from build123d import *

# Parameters (mm, degrees)
F0_W     = 355
F0_H     = 173
F0_R     = 3
F0_R_2   = 2.5
F0_R_3   = 3.25
F1_DEPTH = 20
F2_R     = 4
F3_DEPTH = 20


with BuildPart() as f1:
    # F0 (on Top) → F1 (new body)
    with BuildSketch(Plane.XY):
        with Locations((177.5, 86.5)):
            Rectangle(F0_W, F0_H)
        with Locations((29, 18)):
            Circle(F0_R, mode=Mode.SUBTRACT)
        with Locations((134.5, 72)):
            Circle(F0_R_2, mode=Mode.SUBTRACT)
        with BuildLine():
            Line((206, 13), (198, 13))
            ThreePointArc((198, 13), (196.585786, 13.585786), (196, 15))
            Line((196, 15), (196, 42))
            ThreePointArc((196, 42), (196.585786, 43.414214), (198, 44))
            Line((198, 44), (206, 44))
            ThreePointArc((206, 44), (207.414214, 43.414214), (208, 42))
            Line((208, 42), (208, 15))
            ThreePointArc((208, 15), (207.414214, 13.585786), (206, 13))
        make_face(mode=Mode.SUBTRACT)
        with Locations((269.5, 72)):
            Circle(F0_R_2, mode=Mode.SUBTRACT)
        with Locations((29, 88)):
            Circle(F0_R, mode=Mode.SUBTRACT)
        with BuildLine():
            Line((151.5, 121), (151.5, 71))
            ThreePointArc((151.5, 71), (150.328427, 68.171573), (147.5, 67))
            ThreePointArc((147.5, 67), (144.671573, 68.171573), (143.5, 71))
            Line((143.5, 71), (143.5, 121))
            ThreePointArc((143.5, 121), (144.671573, 123.828427), (147.5, 125))
            ThreePointArc((147.5, 125), (150.328427, 123.828427), (151.5, 121))
        make_face(mode=Mode.SUBTRACT)
        with Locations((134.5, 122)):
            Circle(F0_R_2, mode=Mode.SUBTRACT)
        with Locations((29, 158)):
            Circle(F0_R, mode=Mode.SUBTRACT)
        with BuildLine():
            Line((237, 51), (167, 51))
            ThreePointArc((167, 51), (159.928932, 53.928932), (157, 61))
            Line((157, 61), (157, 131))
            ThreePointArc((157, 131), (159.928932, 138.071068), (167, 141))
            Line((167, 141), (237, 141))
            ThreePointArc((237, 141), (244.071068, 138.071068), (247, 131))
            Line((247, 131), (247, 61))
            ThreePointArc((247, 61), (244.071068, 53.928932), (237, 51))
        make_face(mode=Mode.SUBTRACT)
        with BuildLine():
            ThreePointArc((256.5, 67), (253.671573, 68.171573), (252.5, 71))
            Line((252.5, 71), (252.5, 121))
            ThreePointArc((252.5, 121), (253.671573, 123.828427), (256.5, 125))
            ThreePointArc((256.5, 125), (259.328427, 123.828427), (260.5, 121))
            Line((260.5, 121), (260.5, 71))
            ThreePointArc((260.5, 71), (259.328427, 68.171573), (256.5, 67))
        make_face(mode=Mode.SUBTRACT)
        with Locations((269.5, 122)):
            Circle(F0_R_2, mode=Mode.SUBTRACT)
        with Locations((184.5, 163)):
            Circle(F0_R_3, mode=Mode.SUBTRACT)
        with Locations((219.5, 163)):
            Circle(F0_R_3, mode=Mode.SUBTRACT)
    extrude(amount=F1_DEPTH)

    # F2 (on face) → F3 (cut)
    with BuildSketch(Plane(origin=(0, 0, 0), x_dir=(0, -1, 0), z_dir=(-1, 0, 0))):
        with Locations((-150.5, 10)):
            Circle(F2_R)
        with Locations((-80.5, 10)):
            Circle(F2_R)
        with Locations((-10.5, 10)):
            Circle(F2_R)
    extrude(amount=-F3_DEPTH, mode=Mode.SUBTRACT)


solid = f1.part
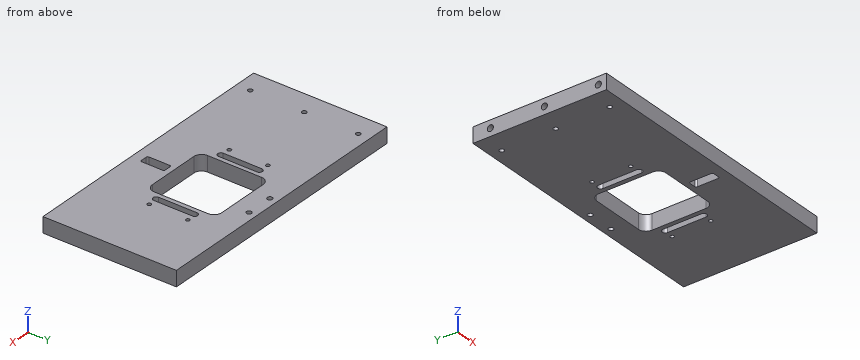
Model file for the job. Use its own axes, mm. Coordinates: 2 decimals unless noted, no trailing zeros. Loops run counter-clockwise (first coordinate to the right, second up) from the corner with the lowest first, then second, coordinate; pieces in that order, holes last. Notation, with made-up numbers: (60.5, 18.5) -> (86.5, 18.5) arc R28 cw to (86.5, 50.5) -> close; hole circle Ø10 at (69, -31). An arc over 180 degrees is marked (long way). Use one line per item in the form item = value. Start each with the question number.
(1) Cut at B-B on z = 3. Give the number of separate pieces and of enclosed holes in the cut face, and give its area (3 significant figures).
(2) Cut at A-A on x = 184.5. Give the cut face in (y, z).
(3) Probe probe 1 along Y at (x, z) = (269.5, 15); probe 2 along Y at (x, z) = (29, 12.75); probe 3 along X at (y, z) = (108.5, 14). List the from-to ranges inside material, lowest first. Write a range as from..to.
(4) Flat gauge pin, fed straight in: pin 1 (4 mm diameter, centred on x = 269.5, y = 122, fed in from -Z). Where does the tip first touch, or does it go through?
Values:
q1.separate_pieces = 1
q1.enclosed_holes = 13
q1.area = 51,900 mm2
q2.outline = (0, 0) -> (51, 0) -> (51, 20) -> (0, 20) -> close; (141, 0) -> (159.75, 0) -> (159.75, 20) -> (141, 20) -> close; (166.25, 0) -> (173, 0) -> (173, 20) -> (166.25, 20) -> close
q3.probe_1 = 0..69.5, 74.5..119.5, 124.5..173
q3.probe_2 = 0..15, 21..85, 91..155, 161..173
q3.probe_3 = 0..143.5, 151.5..157, 247..252.5, 260.5..355
q4.pin_1 = through
